Source: CAD feature listing. Evaluate the final solid. Frame: model axes, mm. A direction names the side the tool comes from. Give positions to 0.01 mm unless a question says otherwise; leave off trailing zeros. Order: outer loops, then holes, each group sorted by start corner. A loop starts at its lowest first (then second) coordinate and runs counter-clockwise, first axis right, second up. Notation, with made-up numbers: (58.25, -17) - (68.25, -17) arc R34 ccw to (68.25, 17) - close; hole circle Ø4 at (-0.5, 1.5). An arc over 180 degrees is marked (long way). Write each question's results on one line, items separated by ' | '. Start each with the question number.
Item 1: Line query: line 1 along Z through (x, y) = (-45, 23); line 2 along X through (y, z) = (21, 4). Output: solid intervals per line, ascending.
Item 2: Section A-A on z = 16.5. Output: boundary loops of the cut face in (x, y).
Item 3: Mould query, pull axis Y, two halves, no side actions, for faces 4 (the cylindrical face through (-47.885, -20.242, 0.796)), 5 (the flat face through (42.88, 21, -2)), 6 (the flat face through (47, 17.48, -2)), 7 (the cylindrical face through (47.365, -20.242, 0.796)). Classes: released by +Y, released by -Y, zero draft, split by the parting line, or undercut.
Item 4: Contact query for flat-ended pins moving along their axis: pin 1 Ø1.8 at (y, z) = (20.5, -2) entering from +X; pin 2 Ø8.5 at (x, y) = (-48, -23.5) entering from -Z; pin 3 Ø3.5 at (x, y) = (47.625, 22.225) entering from +Z; pin 4 Ø8.5 at (x, y) = (-48.5, 22.5) entering from +Z. Output: stop coordinate, or through.
Item 5: Set-up query: faces 1 (the flat face through (-42.88, -21, -2)), 2 (the flat face through (-46, 20.6, 1.57)), 3 (the flat face through (45.9, -20.5, 1.57)). Return all of +Z, -Z, +X, -X, +Y, -Y with unobstructed straight access to the full face (end or side cutting, diameter ignored); none if empty.
```python
from build123d import *

# Parameters (mm, degrees)
SCHIZZO1_W                        = 101.6
SCHIZZO1_H                        = 50.8
ESTRUSIONE_ESTRUSIONE1_DEPTH      = 1.57
SCHIZZO2_R                        = 2
TAGLIO_ESTRUSIONE1_DEPTH          = 57.817822028
ESTRUSIONE_ESTRUSIONE2_DEPTH      = 25.43
ESTRUSIONE_ESTRUSIONE2_DEPTH_BACK = 5.07


with BuildPart() as part:
    # Schizzo1 → Estrusione-Estrusione1 (new body)
    with BuildSketch(Plane.XY):
        Rectangle(SCHIZZO1_W, SCHIZZO1_H)
    extrude(amount=ESTRUSIONE_ESTRUSIONE1_DEPTH)

    # Schizzo2 → Taglio-Estrusione1 (cut, through all)
    with BuildSketch(Plane.XY.offset(1.57)):
        with Locations((-47.625, 22.225)):
            Circle(SCHIZZO2_R)
        with Locations((47.625, 22.225)):
            Circle(SCHIZZO2_R)
        with Locations((47.625, -22.225)):
            Circle(SCHIZZO2_R)
        with Locations((-47.625, -22.225)):
            Circle(SCHIZZO2_R)
    extrude(amount=-TAGLIO_ESTRUSIONE1_DEPTH, mode=Mode.SUBTRACT)

    # Schizzo3 → Estrusione-Estrusione2 (add, two sides: drawn at the far end of the back side and taken through both)
    with BuildSketch(Plane.XY.offset(1.57).offset(-ESTRUSIONE_ESTRUSIONE2_DEPTH_BACK)):
        Polygon((-50.8, 17.48), (-42.88, 17.48), (-42.88, 25.4), (42.88, 25.4), (42.88, 17.48), (50.8, 17.48), (50.8, -17.48), (42.88, -17.48), (42.88, -25.4), (-42.88, -25.4), (-42.88, -17.48), (-50.8, -17.48), align=None)
    extrude(amount=ESTRUSIONE_ESTRUSIONE2_DEPTH + ESTRUSIONE_ESTRUSIONE2_DEPTH_BACK)


solid = part.part
```
Evaluation:
1) line 1: z = 0 to 1.57 | line 2: x = -42.88 to 42.88
2) outline: (-50.8, -17.48) - (-42.88, -17.48) - (-42.88, -25.4) - (42.88, -25.4) - (42.88, -17.48) - (50.8, -17.48) - (50.8, 17.48) - (42.88, 17.48) - (42.88, 25.4) - (-42.88, 25.4) - (-42.88, 17.48) - (-50.8, 17.48) - close
3) face 4: undercut | face 5: zero draft | face 6: released by +Y | face 7: undercut
4) pin 1: stops at x = 42.88 | pin 2: stops at z = 0 | pin 3: passes through | pin 4: stops at z = 1.57
5) face 1: -Z, -X, -Y | face 2: +Z, -X, +Y | face 3: +Z, +X, -Y
